Design review of the part built by this model. Coordinates are the model's own, in mm. Round coordinates to 2 decimals unless told otherwise and drop trailing zeros. Loops run counter-clockwise (first coordinate to the right, second up) from the corner with the lowest first, then second, coordinate; pieces in that order, holes last. Notation, with made-up numbers: M -26.75,9 L 32.25,9 A15 cw 32.25,26 Z; hole C -8.5,-2.75 d5. An arc over 180 degrees is marked long. Use a Markdown table: item, result.
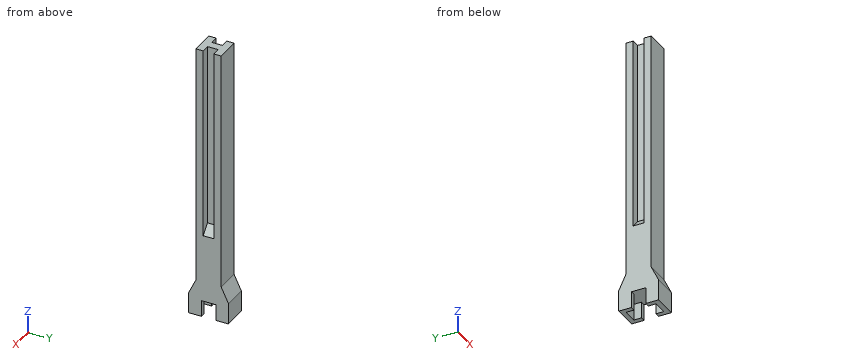
from build123d import *

# Parameters (mm, degrees)
F1_DEPTH  = 6.8
F3_DEPTH  = 2
F3_FACE_W = 10
F3_FACE_H = 16.472
F6_W      = 10
F6_H      = 10.472
F9_DEPTH  = 100
F10_W     = 3.3527343459
F10_H     = 4.472
F11_DEPTH = 20
F13_DEPTH = 4.8


with BuildPart() as f1:
    # F0 (on Top) → F1 (new body)
    with BuildSketch(Plane.XY):
        Polygon((-5, 5.236), (-5, 0), (-3, 0), (-3, 3.236), (0, 3.236), (3, 3.236), (3, 0), (5, 0), (5, 5.236), (0, 5.236), align=None)
    extrude(amount=F1_DEPTH)


with BuildPart() as f1b:
    # F0 (on Top) → F1, piece 2 (new body)
    with BuildSketch(Plane.XY):
        Polygon((-3, -6), (-5, -6), (-5, -11.236), (0, -11.236), (5, -11.236), (5, -6), (3, -6), (3, -9.236), (0, -9.236), (-3, -9.236), align=None)
    extrude(amount=F1_DEPTH)


with BuildPart() as f3:
    # F2 (on face) → F3 (new body)
    with BuildSketch(Plane.XY.offset(6.8)):
        Polygon((-3, 0), (-5, 0), (-5, -11.236), (5, -11.236), (5, 0), (3, 0), (3, 3.236), (-3, 3.236), align=None)
        Polygon((5, 5.236), (-5, 5.236), (-5, 0), (-3, 0), (-3, 3.236), (3, 3.236), (3, 0), (5, 0), align=None)
    extrude(amount=F3_DEPTH)


with BuildPart() as f1_1:
    add(f1.part)

    # F4: union F1b, F3
    add(f1b.part)
    add(f3.part)

    # F3_face (on face) → F7 section 0
    with BuildSketch(Plane(origin=(0, -3, 8.8), x_dir=(1, 0, 0), z_dir=(0, 0, 1))):
        Rectangle(F3_FACE_W, F3_FACE_H)
    # F6 (on offset) → F7 section 1
    with BuildSketch(Plane.XY.offset(15.1)):
        with Locations((0, -3)):
            Rectangle(F6_W, F6_H)
    loft()

    # F8 (on face) → F9 (join)
    with BuildSketch(Plane.XY.offset(15.1)):
        Polygon((5, 2.236), (-5, 2.236), (-5, -0.764), (-1.6472656541, -0.764), (-1.6472656541, -5.236), (-5, -5.236), (-5, -8.236), (5, -8.236), (5, -5.236), (1.6472656541, -5.236), (1.6472656541, -0.764), (5, -0.764), align=None)
    extrude(amount=F9_DEPTH)

    # F10 (on face) → F11 (join)
    with BuildSketch(Plane.XY.offset(15.1)):
        with Locations((3.323632827, -3)):
            Rectangle(F10_W, F10_H)
    extrude(amount=F11_DEPTH)

    # F12 (on face) → F13 (join)
    with BuildSketch(Plane.XZ.offset(0.764)):
        Polygon((1.6472656541, 35.1), (5, 35.1), (1.6472656541, 38.8235887235), align=None)
    extrude(amount=F13_DEPTH)

    # F14: F1 across plane


with BuildPart() as f1_2:
    add(f1_1.part)
    add(f1_1.part.mirror(Plane.YZ))


solid = f1_2.part
1. Insertion check: pin 1 (5 mm diameter, centred on x = -0.5, y = -3.5, fed in from -Z); pin 2 (1.7 mm diameter, centred on x = 4, z = 73.5, fed in from +Y); pin 3 (2.5 mm diameter, centred on x = 4, z = 90.5, fed in from -Y). Each pin has a flat end and moves straight along its axis. Give the tip position at first contact, or say it passes through.
Check values:
| item | result |
|---|---|
| pin 1 | stops at z = 6.8 |
| pin 2 | stops at y = 2.24 |
| pin 3 | stops at y = -8.24 |
2. Take a section at C-C on x = 0.25. Give the boundary of the cut face in (y, z), and give its area (3 significant figures).
Check values:
| item | result |
|---|---|
| outline | M -11.24,0 L -9.24,0 L -9.24,6.8 L 3.24,6.8 L 3.24,0 L 5.24,0 L 5.24,8.8 L 2.24,15.1 L 2.24,115.1 L -8.24,115.1 L -8.24,15.1 L -11.24,8.8 Z |
| area | 1,190 mm² |
3. Take a section at A-A on y = -1.75. Give the boundary of the cut face in (x, z).
Check values:
| item | result |
|---|---|
| outline | M -5,6.8 L 5,6.8 L 5,35.1 L 1.65,38.82 L 1.65,115.1 L -1.65,115.1 L -1.65,38.82 L -5,35.1 Z |
4. Take a section at D-D on z = 24.5. Give the boundary of the cut face in (x, y).
Check values:
| item | result |
|---|---|
| outline | M -5,-8.24 L 5,-8.24 L 5,2.24 L -5,2.24 Z |
5. Wall thickness on line 1 along Y through (x, z) = (3, 110.5); line 2 along Y through (x, z) = (4.75, 31); line 3 along Z through (x, y) = (0, -7): over which ranges is each line inside the solid? List them lowest first. Write a range as from..to.
Check values:
| item | result |
|---|---|
| line 1 | y = -8.24..-5.24, -0.76..2.24 |
| line 2 | y = -8.24..2.24 |
| line 3 | z = 6.8..115.1 |
6. Take a section at B-B on z = 85.5. Give the boundary of the cut face in (x, y).
Check values:
| item | result |
|---|---|
| outline | M -5,-8.24 L 5,-8.24 L 5,-5.24 L 1.65,-5.24 L 1.65,-0.76 L 5,-0.76 L 5,2.24 L -5,2.24 L -5,-0.76 L -1.65,-0.76 L -1.65,-5.24 L -5,-5.24 Z |
